```python
from build123d import *

# Parameters (mm, degrees)
SKETCH_W        = 102
SKETCH_H        = 146
PAD_DEPTH       = 12.9
SKETCH010_R     = 1.5
POCKET_DEPTH    = 102
SKETCH012_R     = 1.5
POCKET005_DEPTH = 5
SKETCH003_W     = 12
SKETCH003_H     = 6
PAD004_DEPTH    = 5.7
SKETCH004_W     = 91
SKETCH004_H     = 10
POCKET007_DEPTH = 0.5


with BuildPart() as part:
    # Sketch → Pad (new body, symmetric)
    with BuildSketch(Plane.XY):
        Rectangle(SKETCH_W, SKETCH_H)
    extrude(amount=PAD_DEPTH, both=True)

    # Sketch010 (on Face3 of Pad) → Pocket (cut)
    with BuildSketch(Plane.YZ.offset(51)):
        with Locations((-52, -7.9)):
            Circle(SKETCH010_R)
        with Locations((8, -7.9)):
            Circle(SKETCH010_R)
        with Locations((38, -7.9)):
            Circle(SKETCH010_R)
    extrude(amount=-POCKET_DEPTH, mode=Mode.SUBTRACT)

    # Sketch012 (on Face3 of Pocket) → Pocket005 (cut)
    with BuildSketch(Plane(origin=(0, 0, -12.9), x_dir=(1, 0, 0), z_dir=(0, 0, -1))):
        with Locations((-47, 42)):
            Circle(SKETCH012_R)
        with Locations((47, 42)):
            Circle(SKETCH012_R)
        with Locations((-47, -28)):
            Circle(SKETCH012_R)
        with Locations((47, -28)):
            Circle(SKETCH012_R)
    extrude(amount=-POCKET005_DEPTH, mode=Mode.SUBTRACT)

    # Sketch003 (on Face2 of Pad) → Pad004 (join)
    with BuildSketch(Plane.XZ.offset(73)):
        with Locations((30, -6.1)):
            Rectangle(SKETCH003_W, SKETCH003_H)
    extrude(amount=PAD004_DEPTH)

    # Sketch004 (on Face2 of Pad) → Pocket007 (cut)
    with BuildSketch(Plane.XZ.offset(73)):
        with Locations((0, 3.6)):
            Rectangle(SKETCH004_W, SKETCH004_H)
    extrude(amount=-POCKET007_DEPTH, mode=Mode.SUBTRACT)


solid = part.part
```
Input: part model. Units: mm. Frame: model coordinates. A direction names the side the tool comes from. Give positions to 0.01 mm unless a question says otherwise; leave off trailing zeros. Order: outer loops, then holes, each group sorted by start corner. A loop starts at its lowest first (then second) coordinate and runs counter-clockwise, first axis right, second up. Notation, with made-up numbers: (38.5, 46) -> (93.5, 46) arc R21 cw to (93.5, 76) -> close; hole circle Ø11 at (3.5, 25). An arc over 180 degrees is marked (long way). Write each question's results on one line, items separated by ' | '. Start each with the question number.
Item 1: Set-up query: faces 5 (the flat face through (30, -76, -9.1)), 6 (the cylindrical face through (0.71, 36.89, -6.89)), 7 (the flat face through (-47, 28, -7.9)), 8 (the flat face through (36, -76, -6)). Return all of +Z, -Z, +X, -X, +Y, -Y with unobstructed straight access to the full face (end or side cutting, diameter ignored); none if empty.
Item 2: Cut plane A-A on x = 17.5. Return the cut outline in (y, z), then the cut area to 3 significant figures.
Item 3: Cut plane C-C on x = -47. Return the cut outline in (y, z), then the cut area to 3 significant figures.
Item 4: Cut plane B-B on y = 8. Return the cut outline in (x, z), then the cut area to 3 significant figures.
Item 5: Contact query for flat-ended pins moving along their axis: P1, Ø1.5, axis at x = -47.5, y = -41.5, coming from the -Z side; P2, Ø1.7, axis at y = -76, z = -6, coming from the -X side; P3, Ø3, axis at x = 30, y = -75.5, coming from the +Z side. Output: stop coordinate, or through.
Item 6: Cut plane D-D on z = 10.5. Return the cut outline in (x, y).
Item 7: Line query: line 1 (X direction, y = 28, z = -11.35); line 2 (Y direction, x = -47, z = -10); line 3 (Z direction, x = 14, y = 8). Output: solid intervals per line, ascending.
Item 8: Mould query, pull axis Y, two halves, no side actions, for faces 1 (the flat face through (47, -42, -7.9)), 2 (the flat face through (-1, 73, 0)), 3 (the flat face through (30, -76, -3.1)), 4 (the cylindrical face through (45.89, 26.99, -10.44)). Classes: pulls with the +Y half, pulls with the -Y half, needs draft (parallel to the pull), parting line crosses it, or undercut.
Established:
1) face 5: -Z, +X, -X, -Y | face 6: +X, -X | face 7: -Z | face 8: +Z, -Z, +X, -Y
2) outline: (-73, -12.9) -> (73, -12.9) -> (73, 12.9) -> (-73, 12.9) -> (-73, 8.6) -> (-72.5, 8.6) -> (-72.5, -1.4) -> (-73, -1.4) -> close; hole circle Ø3 at (-52, -7.9); hole circle Ø3 at (8, -7.9); hole circle Ø3 at (38, -7.9) | area: 3,740 mm^2
3) outline: (-73, -12.9) -> (-43.5, -12.9) -> (-43.5, -7.9) -> (-40.5, -7.9) -> (-40.5, -12.9) -> (26.5, -12.9) -> (26.5, -7.9) -> (29.5, -7.9) -> (29.5, -12.9) -> (73, -12.9) -> (73, 12.9) -> (-73, 12.9) -> close; hole circle Ø3 at (-52, -7.9); hole circle Ø3 at (8, -7.9); hole circle Ø3 at (38, -7.9) | area: 3,720 mm^2
4) outline: (-51, -12.9) -> (51, -12.9) -> (51, -9.4) -> (-51, -9.4) -> close; (-51, -6.4) -> (51, -6.4) -> (51, 12.9) -> (-51, 12.9) -> close | area: 2,330 mm^2
5) P1: z = -7.9 | P2: x = 24 | P3: z = -3.1
6) outline: (-51, -73) -> (51, -73) -> (51, 73) -> (-51, 73) -> close
7) line 1: -51 to -48.5, -45.5 to 45.5, 48.5 to 51 | line 2: -73 to -43.5, -40.5 to 26.5, 29.5 to 73 | line 3: -12.9 to -9.4, -6.4 to 12.9
8) face 1: undercut | face 2: pulls with the +Y half | face 3: needs draft | face 4: undercut
